Check sheet for the modelled part. Datum: model origin and axes. Units: mm. A direction names the side the tool comes from. Round coordinates to 2 decimals unless told otherwise and drop trailing zeros. Write each loop counter-clockwise with the first axis right and the second up, starting at its lowest first coordinate (ties: lowest second). Pieces come first, ordered by that corner, then holes. Notation, with made-up numbers: (9.5, -26) -> (34.5, -26) arc R34 cw to (34.5, 4) -> close; hole circle Ø10 at (31.25, 41). An arc over 180 degrees is marked (long way). One line per item, written item: value.
from build123d import *

# Parameters (mm, degrees)
SKETCH_1_W      = 57
SKETCH_1_H      = 57
SKETCH_1_R      = 2
EXTRUDE_1_DEPTH = 96
SKETCH_2_R      = 4
EXTRUDE_2_DEPTH = 21


with BuildPart() as part:
    # 草圖1 → 填料-伸長1 (new body)
    with BuildSketch(Plane.XY):
        Rectangle(SKETCH_1_W, SKETCH_1_H)
        with Locations((-23.5, 23.5)):
            Circle(SKETCH_1_R, mode=Mode.SUBTRACT)
        with Locations((23.5, 23.5)):
            Circle(SKETCH_1_R, mode=Mode.SUBTRACT)
        with Locations(Location((23.5, -23.5, 0), (0, 0, 180))):
            Circle(SKETCH_1_R, mode=Mode.SUBTRACT)
        with Locations(Location((-23.5, -23.5, 0), (0, 0, 180))):
            Circle(SKETCH_1_R, mode=Mode.SUBTRACT)
    extrude(amount=-EXTRUDE_1_DEPTH)

    # 草圖2 → 填料-伸長2 (add)
    with BuildSketch(Plane.XY):
        with Locations(Location((0, 0, 0), (0, 0, 180))):
            Circle(SKETCH_2_R)
    extrude(amount=EXTRUDE_2_DEPTH)


solid = part.part
Item 1: Mould release check, pull along Y, two halves, no side actions. Record for faces 3 (the flat face through (0, 7, 0)), 4 (the flat face through (0, -28.5, -47)), 5 (the cylindrical face through (-25.1, 22.3, -47.3)), 6 (the flat face through (0, 28.5, -47)): pulls with the +Y half, pulls with the -Y half, needs draft (parallel to the pull), parting line crosses it, or undercut.
Answer:
face 3: needs draft
face 4: pulls with the -Y half
face 5: undercut
face 6: pulls with the +Y half
Item 2: Sectioned sample at C-C on z = -78. Enter the section's corners in (x, y).
Answer:
outline: (-28.5, -28.5) -> (28.5, -28.5) -> (28.5, 28.5) -> (-28.5, 28.5) -> close; hole circle Ø4 at (-23.5, -23.5); hole circle Ø4 at (-23.5, 23.5); hole circle Ø4 at (23.5, -23.5); hole circle Ø4 at (23.5, 23.5)
Item 3: Sectioned sample at D-D on y = 0. Enter the section's corners in (x, z).
Answer:
outline: (-28.5, -96) -> (28.5, -96) -> (28.5, 0) -> (4, 0) -> (4, 21) -> (-4, 21) -> (-4, 0) -> (-28.5, 0) -> close
Item 4: Thickness scan on line 1 (X direction, y = -23.5, z = -23); line 2 (Y direction, x = -23, z = -43); line 3 (Y direction, x = -24.5, z = -83). Record the ranges inside material, lowest first.
Answer:
line 1: x = -28.5 to -25.5, -21.5 to 21.5, 25.5 to 28.5
line 2: y = -28.5 to -25.44, -21.56 to 21.56, 25.44 to 28.5
line 3: y = -28.5 to -25.23, -21.77 to 21.77, 25.23 to 28.5
Item 5: Depth check by flat-ended pin: P1, Ø6, axis at x = -5.5, y = 7, coming from the +Z side; P2, Ø3, axis at x = 23.5, y = 23.5, coming from the -Z side. Enter the tip coordinate at first touch or a pass-through.
Answer:
P1: stops at z = 0
P2: passes through
Item 6: Tool access check on faces 1 (the cylindrical face through (0.867, 3.905, 10.353)), 2 (the flat face through (0, 0, -96)). Record the directions out of +Z, -Z, +X, -X, +Y, -Y that give a thin tool (end or side, any length) a straight path to the whole face; none if there is none.
Answer:
face 1: +Z
face 2: -Z, +X, -X, +Y, -Y
Item 7: Sectioned sample at A-A on x = 23.5. Enter the section's corners in (y, z).
Answer:
outline: (-28.5, -96) -> (-25.5, -96) -> (-25.5, 0) -> (-28.5, 0) -> close; (-21.5, -96) -> (21.5, -96) -> (21.5, 0) -> (-21.5, 0) -> close; (25.5, -96) -> (28.5, -96) -> (28.5, 0) -> (25.5, 0) -> close
